Geometry check sheet. Reference: the model listing, model coordinates, mm. Face numbers are marked on the shaded views. A direction names the side the tool comes from. Give positions to 0.01 mm unless a question says otherwise; leave off trailing zeros. Loops run counter-clockwise (first coordinate to the right, second up) from the corner with the lowest first, then second, coordinate; pieces in that order, holes last. Notation, with made-up numbers: (76, 84) -> (116, 84) arc R37 ccw to (116, 121) -> close; hole circle Ø11 at (-38, 50.25). An arc over 180 degrees is marked (long way). Write item = value, one per line. Start each with the question number.
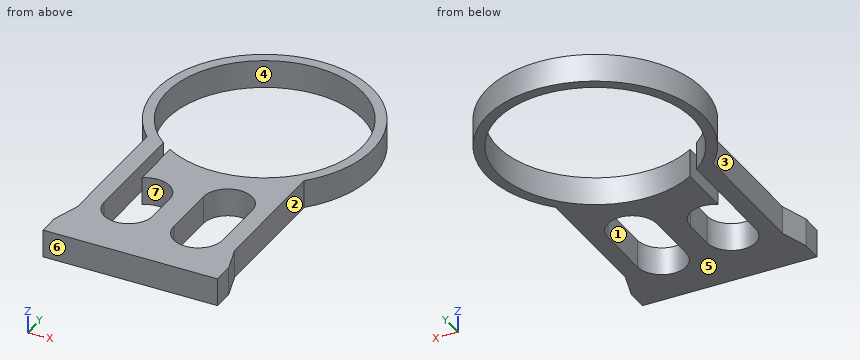
```python
from build123d import *

# Parameters (mm, degrees)
DODANIE_WYCI_GNI_CIE1_DEPTH = 4


with BuildPart() as part:
    # Szkic1 → Dodanie-wyciągnięcie1 (new body)
    with BuildSketch(Plane.XY):
        with BuildLine():
            Line((12.5, 0), (-12.5, 0))
            Line((-12.5, 0), (-12.5, 3))
            Line((-12.5, 3), (-11.25, 7))
            Line((-11.25, 7), (-11.25, 25.837565944))
            ThreePointArc((-11.25, 25.837565944), (0, 52), (11.25, 25.837565944))
            Line((11.25, 25.837565944), (11.25, 7))
            Line((11.25, 7), (12.5, 3))
            Line((12.5, 3), (12.5, 0))
        make_face()
        with BuildLine():
            Line((8.75, 16.5), (8.75, 8.5))
            ThreePointArc((8.75, 8.5), (5.25, 5), (1.75, 8.5))
            Line((1.75, 8.5), (1.75, 16.5))
            ThreePointArc((1.75, 16.5), (5.25, 20), (8.75, 16.5))
        make_face(mode=Mode.SUBTRACT)
        with BuildLine():
            Line((-1.75, 14), (-1.75, 9.5))
            ThreePointArc((-1.75, 9.5), (-5.25, 6), (-8.75, 9.5))
            Line((-8.75, 9.5), (-8.75, 14))
            Line((-8.75, 14), (-8.75, 25.571253503))
            ThreePointArc((-8.75, 25.571253503), (8.017135871, 47.977174409), (-7.25, 24.523460433))
            Line((-7.25, 24.523460433), (-7.25, 16.872281323))
            ThreePointArc((-7.25, 16.872281323), (-3.629814825, 17.102418411), (-1.75, 14))
        make_face(mode=Mode.SUBTRACT)
    extrude(amount=DODANIE_WYCI_GNI_CIE1_DEPTH)


solid = part.part
```
1) Section check A-A (y = 36.5). Enter the section's corners in (x, z), plus the area to 3 significant figures.
2) Section check C-C (z = 3.3). Enter the section's corners in (x, y), plus the area to 3 significant figures.
3) Thickness scan on line 1 (X direction, y = 36.5, z = 3.1); line 2 (X direction, y = 14, z = 1.7); line 3 (Y direction, x = -5.5, z = 0.85). Record the ranges inside material, lowest first.
4) Tool access check on the marked faces 1, 2 and 3. Record the directions out of +Z, -Z, +X, -X, +Y, -Y that give a thin tool (end or side, any length) a straight path to the whole face; none if there is none.
5) Section check D-D (x = 5.25). Enter the section's corners in (y, z).
6) Draft check along Y on the marked faces 4, 5, 6 and 7. Enter one of: released by +Y, released by -Y, zero draft, split by the parting line, or undercut.
7) Depth check by flat-ended pin: pin 1 Ø2 at (y, z) = (15, 2) entering from -X; pin 2 Ø8 at (x, y) = (9, 17.5) entering from -Z; pin 3 Ø1.5 at (y, z) = (1.5, 3) entering from +X. Enter the tip coordinate at first touch or a pass-through.
8) Section check B-B (x = 0). Enter the section's corners in (y, z), plus the area to 3 significant figures.
Check result:
q1.outline = (-15.5, 0) -> (-14, 0) -> (-14, 4) -> (-15.5, 4) -> close; (14, 0) -> (15.5, 0) -> (15.5, 4) -> (14, 4) -> close
q1.area = 12.0 mm2
q2.outline = (-12.5, 0) -> (12.5, 0) -> (12.5, 3) -> (11.25, 7) -> (11.25, 25.84) arc R15.5 ccw (long way) to (-11.25, 25.84) -> (-11.25, 7) -> (-12.5, 3) -> close; hole (-8.75, 9.5) arc R3.5 ccw to (-1.75, 9.5) -> (-1.75, 14) arc R3.5 ccw to (-7.25, 16.87) -> (-7.25, 24.52) arc R14 ccw (long way) to (-8.75, 25.57) -> close; hole (1.75, 8.5) arc R3.5 ccw to (8.75, 8.5) -> (8.75, 16.5) arc R3.5 ccw to (1.75, 16.5) -> close
q2.area = 480 mm2
q3.line_1 = -15.5 to -14, 14 to 15.5
q3.line_2 = -11.25 to -8.75, -1.75 to 1.75, 8.75 to 11.25
q3.line_3 = 0 to 6.01, 17.49 to 23.63, 49.37 to 50.99
q4.face_1 = +Z, -Z
q4.face_2 = +Z, -Z, +X
q4.face_3 = +Z, -Z, -X
q5.outline = (0, 0) -> (5, 0) -> (5, 4) -> (0, 4) -> close; (20, 0) -> (23.52, 0) -> (23.52, 4) -> (20, 4) -> close; (49.48, 0) -> (51.08, 0) -> (51.08, 4) -> (49.48, 4) -> close
q6.face_4 = undercut
q6.face_5 = zero draft
q6.face_6 = released by -Y
q6.face_7 = undercut
q7.pin_1 = -11.25
q7.pin_2 = 0
q7.pin_3 = 12.5
q8.outline = (0, 0) -> (22.5, 0) -> (22.5, 4) -> (0, 4) -> close; (50.5, 0) -> (52, 0) -> (52, 4) -> (50.5, 4) -> close
q8.area = 96.0 mm2
